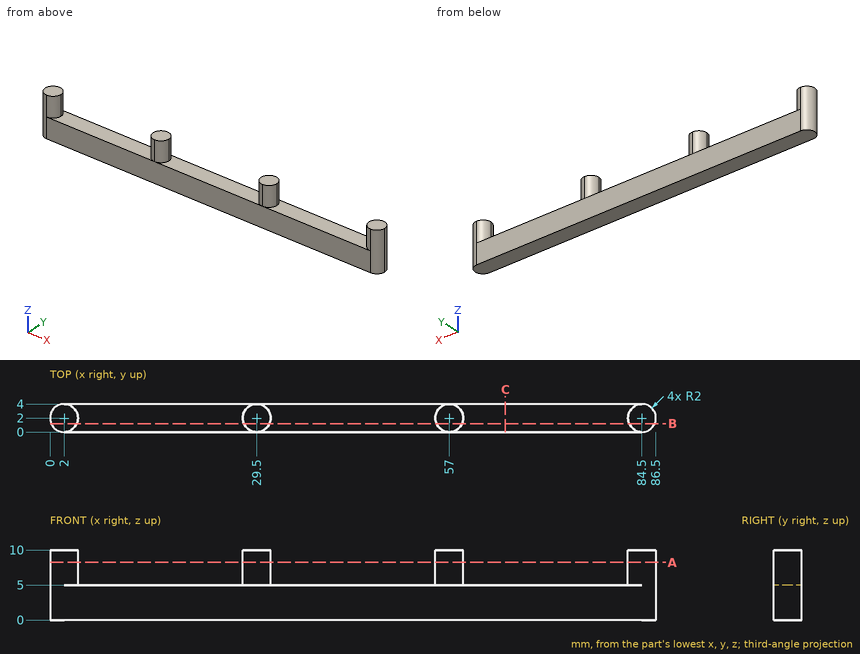
Geometry: see drawing. Coordinates: mm, zero at the bounding-box minimum. Round coordinates to 2 decimals unless told otherwise and drop trailing zeros. Loops run counter-clockwise (first coordinate to the right, second up) from the corner with the lowest first, then second, coordinate; pieces in that order, holes last. Notation, with made-up numbers: (0, 81) - (57, 81) arc R23 ccw to (57, 90) - close; hole circle Ø11 at (42.5, -15.5). An arc over 180 degrees is marked (long way). Write item = value, one per line. Start each with the question number.
(1) Pin query (flat end, axial travel): pin 1 (2 mm diameter, centred on x = 44, y = 3, fed in from +Z); pin 2 (1.5 mm diameter, centred on y = 1, z = 3.5, fed in from +X); pin 3 (2 mm diameter, centred on y = 3, z = 7, fed in from -X). Return the tip coordinate at first contact, or that it passes through.
(2) Section query A-A, the plane z = 8.25. Output: boundary loops of the cut face in (x, y), plus the area to 3 significant figures.
(3) Section query B-B, the plane y = 1.2. Output: boundary loops of the cut face in (x, z), plus the area to 3 significant figures.
(4) Section query C-C, the plane x = 65. Output: boundary loops of the cut face in (y, z), plus the area to 3 significant figures.
(5) Ray query, line 1 along X through (y, z) = (1.8, 8.25); line 2 along X through (y, z) = (1.15, 6.5); line 3 along Z through (x, y) = (66, 3). Return the intervals inside material, ascending. Write a range as from..to.
Conclusion:
q1.pin_1 = 5
q1.pin_2 = 86.48
q1.pin_3 = 0
q2.outline = (2, 0) arc R2 ccw to (4, 2) arc R2 ccw to (2, 4) arc R2 ccw to start; (27.5, 2) arc R2 ccw to (29.5, 0) arc R2 ccw to (31.5, 2) arc R2 ccw to (29.5, 4) arc R2 ccw to start; (55, 2) arc R2 ccw to (57, 0) arc R2 ccw to (59, 2) arc R2 ccw to (57, 4) arc R2 ccw to start; (82.5, 2) arc R2 ccw to (84.5, 0) arc R2 ccw to (86.5, 2) arc R2 ccw to (84.5, 4) arc R2 ccw to start
q2.area = 50.3 mm2
q3.outline = (0.17, 0) - (86.33, 0) - (86.33, 10) - (82.67, 10) - (82.67, 5) - (58.83, 5) - (58.83, 10) - (55.17, 10) - (55.17, 5) - (31.33, 5) - (31.33, 10) - (27.67, 10) - (27.67, 5) - (3.83, 5) - (3.83, 10) - (0.17, 10) - close
q3.area = 504 mm2
q4.outline = (0, 0) - (4, 0) - (4, 5) - (0, 5) - close
q4.area = 20.0 mm2
q5.line_1 = 0.01..3.99, 27.51..31.49, 55.01..58.99, 82.51..86.49
q5.line_2 = 0.19..3.81, 27.69..31.31, 55.19..58.81, 82.69..86.31
q5.line_3 = 0..5
